Geometry check sheet. Reference: the model listing, model coordinates, mm. A direction names the side the tool comes from. Coordinates: 2 decimals unless noted, no trailing zeros. Order: outer loops, then holes, each group sorted by start corner. A loop starts at its lowest first (then second) coordinate and runs counter-clockwise, first axis right, second up. Notation, with made-up numbers: (-28, 40) -> (11, 40) arc R14 ccw to (11, 57) -> close; hole circle Ø3 at (7, 0). An arc over 180 degrees is marked (long way). Answer in a Markdown table with one row per item. Add a question column.
```python
from build123d import *

# Parameters (mm, degrees)
ESQUISSE1_W                = 60
ESQUISSE1_H                = 120
BOSS_EXTRU_1_DEPTH         = 20
ENL_V_MAT_EXTRU_1_DEPTH    = 61
ESQUISSE3_W                = 16
ESQUISSE3_H                = 10
ENL_V_MAT_EXTRU_3_DEPTH    = 5
ESQUISSE4_R                = 10
ENL_V_MAT_EXTRU_4_DEPTH    = 21
ESQUISSE5_R                = 1
ENL_V_MAT_EXTRU_5_DEPTH    = 20
R_P_TITION_LIN_AIRE1_COUNT = 3
R_P_TITION_LIN_AIRE1_PITCH = 10
R_P_TITION_LIN_AIRE2_COUNT = 3
R_P_TITION_LIN_AIRE2_PITCH = 10


with BuildPart() as part:
    # Esquisse1 → Boss.-Extru.1 (new body)
    with BuildSketch(Plane.XY):
        with Locations((38.463255814, 60)):
            Rectangle(ESQUISSE1_W, ESQUISSE1_H)
    extrude(amount=BOSS_EXTRU_1_DEPTH)

    # Esquisse2 → Enlèv. mat.-Extru.1 (cut, through all)
    with BuildSketch(Plane(origin=(68.463255814, 0, 0), x_dir=(0, 0, -1), z_dir=(1, 0, 0))):
        Polygon((-20, 110), (-16, 110), (-16, 115), (-4, 115), (-4, 5), (-16, 5), (-16, 10), (-20, 10), align=None)
    extrude(amount=-ENL_V_MAT_EXTRU_1_DEPTH, mode=Mode.SUBTRACT)

    # Esquisse3 → Enlèv. mat.-Extru.3 (cut)
    with BuildSketch(Plane(origin=(0, 120, 0), x_dir=(1, 0, 0), z_dir=(0, 1, 0))):
        with Locations((38.463255814, -10)):
            Rectangle(ESQUISSE3_W, ESQUISSE3_H)
    extrude(amount=-ENL_V_MAT_EXTRU_3_DEPTH, mode=Mode.SUBTRACT)

    # Esquisse4 → Enlèv. mat.-Extru.4 (cut, through all)
    with BuildSketch(Plane(origin=(0, 0, 0), x_dir=(-1, 0, 0), z_dir=(0, 0, -1))):
        with Locations((-38.463255814, 28)):
            Circle(ESQUISSE4_R)
    extrude(amount=-ENL_V_MAT_EXTRU_4_DEPTH, mode=Mode.SUBTRACT)

    # Esquisse5 → Enlèv. mat.-Extru.5 (cut)
    with BuildSketch(Plane.XZ):
        with Locations((38.463255814, 18)):
            Circle(ESQUISSE5_R)
        with Locations((38.463255814, 2)):
            Circle(ESQUISSE5_R)
        with Locations((38.463255814, 10)):
            Circle(ESQUISSE5_R)
    enl_v_mat_extru_5 = extrude(amount=-ENL_V_MAT_EXTRU_5_DEPTH, mode=Mode.SUBTRACT)

    # Répétition linéaire1: Enlèv. mat.-Extru.5 ×3
    with Locations(*[(i * R_P_TITION_LIN_AIRE1_PITCH, 0, 0) for i in range(1, R_P_TITION_LIN_AIRE1_COUNT)]):
        add(enl_v_mat_extru_5, mode=Mode.SUBTRACT)

    # Répétition linéaire2: Enlèv. mat.-Extru.5 ×3
    with Locations(*[(-i * R_P_TITION_LIN_AIRE2_PITCH, 0, 0) for i in range(1, R_P_TITION_LIN_AIRE2_COUNT)]):
        add(enl_v_mat_extru_5, mode=Mode.SUBTRACT)


solid = part.part
```
(1) Cross-section at A-A (z = 7). Enter the section's corners in (x, y).
(2) Go/stop test with flat-tipped pins: P1, Ø1.5, axis at x = 17.5, y = 66, coming from the -Z side; P2, Ø1, axis at x = 18.5, z = 2, coming from the -Y side; P3, Ø12, axis at x = 38.46, y = 28, coming from the -Z side; P4, Ø1, axis at x = 28, y = 27.5, coming from the +Z side. Record where each tip stops, or that it passes through.
(3) Access from +Z, -Z, +X, -X, +Y, -Y to the whole of each face (thin tool, end or side, straight path). Record for faces 4 (the face through (38, 0, 8)), 5 (the face through (46.399, 21.915, 1.972)), 6 (the face through (46.463, 118, 10)), 7 (the face through (39, 110, 18)), 8 (the face through (39, 112, 16)).
(4) Scan lines: line 1 along Z through (x, y) = (54, 111); line 2 along Y through (x, z) = (54, 11.75); line 3 along Z through (x, y) = (32, 39). Record each from-to range of solid material in increasing order.
(5) Mould release check, pull along X, two halves, no side actions. Record for faces 1 (the face through (38, 115, 20)), 2 (the face through (68.463, 60, 3)), 3 (the face through (30.463, 118, 10)): +X half, -X half, draft (parallel to the pull), parting line (faces both ways), or undercut.
(6) Cross-section at D-D (x = 13.5). Enter the section's corners in (y, z), plus the area to 3 significant figures.
(7) Cross-section at B-B (y = 28). Enter the section's corners in (x, z).
(8) Cross-section at C-C (x = 42). Enter the section's corners in (y, z).
Checks:
| question | item | result |
|---|---|---|
| 1 | outline | (8.46, 0) -> (68.46, 0) -> (68.46, 5) -> (8.46, 5) -> close; (8.46, 115) -> (30.46, 115) -> (30.46, 120) -> (8.46, 120) -> close; (46.46, 115) -> (68.46, 115) -> (68.46, 120) -> (46.46, 120) -> close |
| 2 | P1 | z = 0 |
| 2 | P2 | y = 20 |
| 2 | P3 | through |
| 2 | P4 | z = 4 |
| 3 | face 4 | +Z, -Z, +X, -X, -Y |
| 3 | face 5 | +Z, -Z |
| 3 | face 6 | +Y |
| 3 | face 7 | +Z, +X, -X |
| 3 | face 8 | +X, -X |
| 4 | line 1 | 0 to 4, 16 to 20 |
| 4 | line 2 | 0 to 5, 115 to 120 |
| 4 | line 3 | 0 to 4 |
| 5 | face 1 | draft |
| 5 | face 2 | +X half |
| 5 | face 3 | undercut |
| 6 | outline | (0, 0) -> (120, 0) -> (120, 20) -> (110, 20) -> (110, 16) -> (115, 16) -> (115, 4) -> (5, 4) -> (5, 16) -> (10, 16) -> (10, 20) -> (0, 20) -> close |
| 6 | area | 680 mm² |
| 7 | outline | (8.46, 0) -> (28.46, 0) -> (28.46, 4) -> (8.46, 4) -> close; (48.46, 0) -> (68.46, 0) -> (68.46, 4) -> (48.46, 4) -> close |
| 8 | outline | (0, 0) -> (18.65, 0) -> (18.65, 4) -> (5, 4) -> (5, 16) -> (10, 16) -> (10, 20) -> (0, 20) -> close; (37.35, 0) -> (120, 0) -> (120, 5) -> (115, 5) -> (115, 4) -> (37.35, 4) -> close; (110, 16) -> (115, 16) -> (115, 15) -> (120, 15) -> (120, 20) -> (110, 20) -> close |
